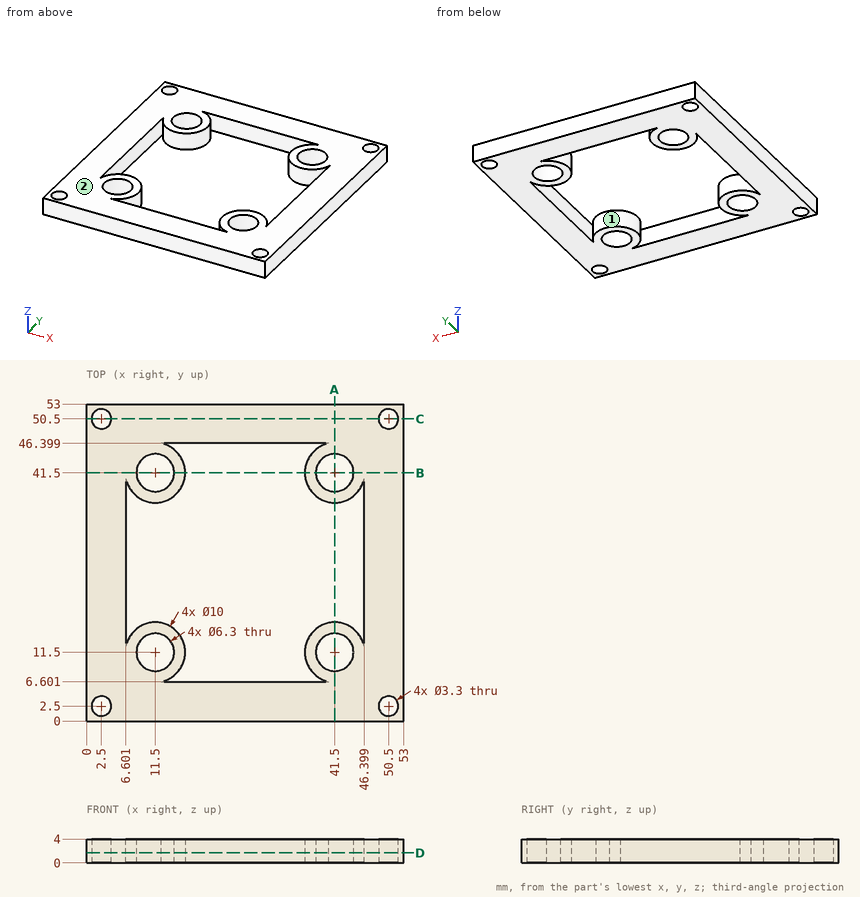
Input: dimensioned drawing with shaded views. Units: mm. Origin: part minimum x, y, z. Coordinates: 2 decimals unless noted, no trailing zeros. Loops run counter-clockwise (first coordinate to the right, second up) from the corner with the lowest first, then second, coordinate; pieces in that order, holes last. Notation, with made-up numbers: (-27.5, -27) -> (18.5, -27) arc R16 cw to (18.5, -18) -> close; hole circle Ø11 at (-21.75, -33). An arc over 180 degrees is marked (long way). Use a Markdown table: item, result. Add a question column.
(1) Section query D-D, the plane z = 1.7. State how many separate pieces and enclosed holes the cut face has, plus the area to 3 significant figures.
(2) Pin query (flat end, axial travel): pin 1 Ø4.5 at (x, y) = (50.5, 2.5) entering from -Z. Return the tip coordinate at first contact, or that it passes through.
(3) Section query C-C, the plane y = 50.5. Return loops of the section in (x, z), plus the area to 3 significant figures.
(4) Mould query, pull axis X, two halves, no side actions, for the marked faces 1 and 2. Classes: pulls with the +X half, pulls with the -X half, needs draft (parallel to the pull), parting line crosses it, or undercut.
(5) Line query: line 1 along Y through (x, z) = (11.5, 1.9); line 2 along Y through (x, z) = (2.5, 2.8); line 3 along Y through (x, z) = (31, 0.8). Output: solid intervals per line, ascending.
(6) Section query A-A, the plane x = 41.5. Return loops of the section in (y, z).
Answer:
| question | item | result |
|---|---|---|
| 1 | separate pieces | 1 |
| 1 | enclosed holes | 9 |
| 1 | area | 1,400 mm^2 |
| 2 | pin 1 | stops at z = 0 |
| 3 | outline | (0, 0) -> (0.85, 0) -> (0.85, 4) -> (0, 4) -> close; (4.15, 0) -> (48.85, 0) -> (48.85, 4) -> (4.15, 4) -> close; (52.15, 0) -> (53, 0) -> (53, 4) -> (52.15, 4) -> close |
| 3 | area | 186 mm^2 |
| 4 | face 1 | undercut |
| 4 | face 2 | needs draft |
| 5 | line 1 | y = 0 to 8.35, 14.65 to 16.5, 36.5 to 38.35, 44.65 to 53 |
| 5 | line 2 | y = 0 to 0.85, 4.15 to 48.85, 52.15 to 53 |
| 5 | line 3 | y = 0 to 6.6, 46.4 to 53 |
| 6 | outline | (0, 0) -> (8.35, 0) -> (8.35, 4) -> (0, 4) -> close; (14.65, 0) -> (16.5, 0) -> (16.5, 4) -> (14.65, 4) -> close; (36.5, 0) -> (38.35, 0) -> (38.35, 4) -> (36.5, 4) -> close; (44.65, 0) -> (53, 0) -> (53, 4) -> (44.65, 4) -> close |
